For this review, take the finished solid that the model builds, in its own axes (mm). A direction names the side the tool comes from. Round coordinates to 2 decimals unless told otherwise and drop trailing zeros. One line per question, with ' | ' between items.
```python
from build123d import *

# Parameters (mm, degrees)
F0_R     = 55
F1_DEPTH = 10
F2_R     = 1
F3_R     = 51
F3_R_2   = 50
F4_DEPTH = 4
F5_R     = 2


with BuildPart() as f1:
    # F0 (on Top) → F1 (new body)
    with BuildSketch(Plane.XY):
        Circle(F0_R)
    extrude(amount=F1_DEPTH)

    # F2
    f2_edges = [f1.edges().sort_by_distance(p)[0] for p in [
        (-55, 0, 0),
    ]]
    fillet(f2_edges, radius=F2_R)

    # F3 (on face) → F4 (cut)
    with BuildSketch(Plane(origin=(0, 0, 0), x_dir=(1, 0, 0), z_dir=(0, 0, -1))):
        Circle(F3_R)
        Circle(F3_R_2, mode=Mode.SUBTRACT)
    extrude(amount=-F4_DEPTH, mode=Mode.SUBTRACT)

    # F5
    f5_edges = [f1.edges().sort_by_distance(p)[0] for p in [
        (-55, 0, 10),
    ]]
    fillet(f5_edges, radius=F5_R)


solid = f1.part
```
(1) For faces 4 (the flat face through (-1, 1, 10)), 5 (the cylindrical face through (47.69, -15.02, 1.97)), list the 3-axis set-ups (+Z, -Z, +X, -X, +Y, -Y) from which the entire face can be reached by the end or side of a thin tool; tool diameter is ignored.
Output values:
face 4: +Z, +X, -X, +Y, -Y | face 5: -Z
(2) Insertion check: pin 1 (1.5 mm diameter, centred on x = -34.5, z = 5.5, fed in from +Y); pin 2 (3 mm diameter, centred on x = 4.5, z = 6.5, fed in from -Y); pin 3 (6 mm diameter, centred on x = -20, z = 3.5, fed in from +Y). Each pin has a flat end and moves straight along its axis. Give the tip position at first contact, or say it passes through.
Output values:
pin 1: y = 43.43 | pin 2: y = -54.92 | pin 3: y = 52.31
(3) Mouldability with a two-part tool opening along X and no side actions: class faces 1 (the flat face through (33.8, 37.5, 4)), 2 (the cylindrical face through (-11.923, -53.692, 4.451)), 3 (the flat face through (-1, 1, 0)) as released by +X, released by -X, zero draft, split by the parting line, or undercut.
Output values:
face 1: undercut | face 2: split by the parting line | face 3: zero draft
(4) For probe 1 along Y at (x, z) = (0, 1.95); probe 2 along X at (y, z) = (31.5, 1.75); probe 3 along X at (y, z) = (10.5, 2.75), list the stretches that pass through material, from the lowest coordinate up. Write a range as [from, to].
Output values:
probe 1: [-55, -51], [-50, 50], [51, 55] | probe 2: [-45.09, -40.11], [-38.83, 38.83], [40.11, 45.09] | probe 3: [-53.99, -49.91], [-48.89, 48.89], [49.91, 53.99]
